Geometry: final body of the model. Coordinates: model frame, mm. A direction names the side the tool comes from. Coordinates: 2 decimals unless noted, no trailing zeros. Write each loop counter-clockwise with the first axis right and the second up, starting at its lowest first coordinate (ties: lowest second). Pieces come first, ordered by that corner, then holes. Notation, with made-up numbers: M 51.25,-3.75 L 101.25,-3.75 A18 ccw 101.25,26.25 Z; hole C 27.5,-16.5 d4. An arc over 180 degrees is marked long. Write item = value, one per line. Start each with the question number.
Item 1: Section B-B on z = -15. Output: boundary loops of the cut face in (x, y).
Item 2: Pull-direction query (Z, two-part tool) for faces 3 (the cylindrical face through (47.69, -69.02, 15.02)), 4 (the cylindrical face through (-1.302, -60.56, 13.113)), 5 (the flat face through (22, -140, -22)), 6 (the cylindrical face through (-29.97, -120.28, 1.32)); classes: +Z half, -Z half, draft (parallel to the pull), parting line (faces both ways), or undercut.
Item 3: Reachability of faces 1 (the flat face through (6, -100, -6)), 2 (the flat face through (-1, 0, 1)) from +Z, -Z, +X, -X, +Y, -Y: full face, straight path, thin tool, end or side. Return the list, or none.
Item 4: Section C-C on y = -113. Output: boundary loops of the cut face in (x, z), plus the area to 3 significant figures.
Item 5: First-contact query: pin 1 Ø8 at (x, z) = (14.5, -19.5) entering from -Y; pin 2 Ø5 at (y, z) = (-92.5, -32.5) entering from +X; pin 3 Ø1 at (y, z) = (-35.5, -29.5) entering from +X; pin 4 Ø10 at (x, z) = (-10.5, -26.5) entering from -Y. Flat tips, straight axial feed; report the tip coordinate or a pass-through.
Item 6: Section A-A on x = 0. Output: boundary loops of the cut face in (y, z), plus the area to 3 significant figures.
Item 7: Section D-D on y = -13.5. Output: boundary loops of the cut face in (x, z), plus the area to 3 significant figures.
Item 8: Ray query, L1, parallel to Z at x = 0, y = -108.5; L2, parallel to Z at x = 0, y = -49.5; L3, parallel to Y at x = 16, z = -4. Return the intervals inside material, ascending. Write a range as [from, to].
from build123d import *

# Parameters (mm, degrees)
F0_R     = 50
F1_DEPTH = 140
F2_R     = 30
F3_DEPTH = 40
F4_R     = 10
F5_DEPTH = 80


with BuildPart() as f1:
    # F0 (on Front) → F1 (new body)
    with BuildSketch(Plane.XZ):
        Circle(F0_R)
    extrude(amount=F1_DEPTH)

    # F2 (on face) → F3 (cut)
    with BuildSketch(Plane.XZ.offset(140)):
        Circle(F2_R)
    extrude(amount=-F3_DEPTH, mode=Mode.SUBTRACT)

    # F4 (on face) → F5 (cut)
    with BuildSketch(Plane.XZ.offset(100)):
        with Locations((0, 3.197924)):
            Circle(F4_R)
    extrude(amount=-F5_DEPTH, mode=Mode.SUBTRACT)


solid = f1.part
Responses:
q1.outline = M -47.7,-140 L -25.98,-140 L -25.98,-100 L 25.98,-100 L 25.98,-140 L 47.7,-140 L 47.7,0 L -47.7,0 Z
q2.face_3 = parting line
q2.face_4 = undercut
q2.face_5 = draft
q2.face_6 = undercut
q3.face_1 = -Y
q3.face_2 = +Z, -Z, +X, -X, +Y
q4.outline = C 0,0 d100; hole C 0,0 d60
q4.area = 5,030 mm²
q5.pin_1 = -100
q5.pin_2 = 40
q5.pin_3 = 40.73
q5.pin_4 = -140
q6.outline = M -140,-50 L 0,-50 L 0,50 L -140,50 L -140,30 L -100,30 L -100,13.2 L -20,13.2 L -20,-6.8 L -100,-6.8 L -100,-30 L -140,-30 Z
q6.area = 10,000 mm²
q7.outline = C 0,0 d100
q7.area = 7,850 mm²
q8.L1 = [-50, -30], [30, 50]
q8.L2 = [-50, -6.8], [13.2, 50]
q8.L3 = [-100, 0]
